Geometry check sheet. Reference: the model listing, model coordinates, mm. A direction names the side the tool comes from. Round coordinates to 2 decimals unless told otherwise and drop trailing zeros. Loops run counter-clockwise (first coordinate to the right, second up) from the corner with the lowest first, then second, coordinate; pieces in that order, holes last. Notation, with made-up numbers: M 55,37 L 91,37 A22 ccw 91,45 Z; hole C 10.5,25 d9. An arc over 180 degrees is marked long. Use one line per item in the form item = value. Start each with the question number.
1. Material ranges on line 1 (Z direction, x = -14, y = -122); line 2 (Z direction, x = -56, y = -116.5); line 3 (Z direction, x = 24.5, y = -119), recorded low to high.
2. Cross-section at C-C (z = 9.5). Record the boundary of the cut face in (x, y).
3. Cross-section at D-D (z = 34.5). Record the boundary of the cut face in (x, y).
4. Cross-section at B-B (y = -124). State how many separate pieces and enclosed holes the cut face has, then the cut area to 3 significant figures.
5. Go/stop test with flat-tipped pins: pin 1 (1 mm diameter, centred on x = 19, z = 45.5, fed in from +Y); pin 2 (10 mm diameter, centred on x = -14.5, z = 44.5, fed in from -Y); pin 3 (10 mm diameter, centred on x = -21, z = 31.5, fed in from -Y). Record where each tip stops, or that it passes through.
6. Cross-section at A-A (z = 44). Record the boundary of the cut face in (x, y), then the cut area to 3 significant figures.
7. Draft check along Z on faces 1 (the flat face through (-1, -124, 37.5)), 2 (the flat face through (-65.03, -108, 46)), 3 (the flat face through (-1, -116, 66)), 4 (the flat face through (-1, -112.1, 52)). Enter one of: pulls with the +Z half, pulls with the -Z half, needs draft (parallel to the pull), parting line crosses it, or undercut.
8. Set-up check for faces 5 (the flat face through (64.97, -108, 46)), 6 (the cylindrical face through (-0.995, -137.496, 38.966)), 7 (the flat face through (-1, -122, 40.46)), 8 (the cylindrical face through (-0.995, -122.496, 16.96)): record each of +Z, -Z, +X, -X, +Y, -Y from which the full face is reachable in a straight line by a thin tool's end or side.
```python
from build123d import *

# Parameters (mm, degrees)
BOX003_W      = 570
BOX003_H      = 100
BOX003_DEPTH  = 22.5
TUBE003_R     = 250
TUBE003_R_2   = 122.5
TUBE003_DEPTH = 37.5
TUBE002_R     = 250
TUBE002_R_2   = 122.5
TUBE002_DEPTH = 37.5
TUBE001_R     = 250
TUBE001_R_2   = 122.5
TUBE001_DEPTH = 40.5
BOX001_W      = 570
BOX001_H      = 100
BOX001_DEPTH  = 22.5
BOX_W         = 130
BOX_H         = 70
BOX_DEPTH     = 72
FILLET_R      = 1
FILLET001_R   = 0.5
FILLET002_R   = 0.5
FILLET003_R   = 0.5


with BuildPart() as sphere:
    # Sphere → Sphere (revolve)
    with BuildSketch(Plane(origin=(-0.01, -10.37, -8.39), x_dir=(1, 0, 0), z_dir=(0, -1, 0))):
        with BuildLine():
            ThreePointArc((0, -110), (110, 0), (0, 110))
            Line((0, 110), (0, -110))
        make_face()
    revolve(axis=Axis((-0.01, -10.37, -8.39), (0, 0, 1)))


with BuildPart() as box003:
    # Box003 → Box003 (new body)
    with BuildSketch(Plane(origin=(-285.31, -232.1, 44.4), x_dir=(1, 0, 0), z_dir=(0, 0, 1))):
        with Locations((285, 50)):
            Rectangle(BOX003_W, BOX003_H)
    extrude(amount=BOX003_DEPTH)


with BuildPart() as tube003:
    # Tube003 → Tube003 (new body)
    with BuildSketch(Plane(origin=(0, -15, 10), x_dir=(1, 0, 0), z_dir=(0, 0, 1))):
        Circle(TUBE003_R)
        Circle(TUBE003_R_2, mode=Mode.SUBTRACT)
    extrude(amount=TUBE003_DEPTH)


with BuildPart() as tube002:
    # Tube002 → Tube002 (new body)
    with BuildSketch(Plane(origin=(0, -5, -10), x_dir=(1, 0, 0), z_dir=(0, 0, 1))):
        Circle(TUBE002_R)
        Circle(TUBE002_R_2, mode=Mode.SUBTRACT)
    extrude(amount=TUBE002_DEPTH)


with BuildPart() as tube001:
    # Tube001 → Tube001 (new body)
    with BuildSketch(Plane.XY.offset(-3)):
        Circle(TUBE001_R)
        Circle(TUBE001_R_2, mode=Mode.SUBTRACT)
    extrude(amount=TUBE001_DEPTH)


with BuildPart() as box001:
    # Box001 → Box001 (new body)
    with BuildSketch(Plane(origin=(-285.31, -212.1, 40.46), x_dir=(1, 0, 0), z_dir=(0, 0, 1))):
        with Locations((285, 50)):
            Rectangle(BOX001_W, BOX001_H)
    extrude(amount=BOX001_DEPTH)


with BuildPart() as fillet003:
    # Box → Box (new body)
    with BuildSketch(Plane(origin=(-65.03, -170.42, -6), x_dir=(1, 0, 0), z_dir=(0, 0, 1))):
        with Locations((65, 35)):
            Rectangle(BOX_W, BOX_H)
    extrude(amount=BOX_DEPTH)

    # Cut: cut Box001
    add(box001.part, mode=Mode.SUBTRACT)

    # Cut001: cut Tube001
    add(tube001.part, mode=Mode.SUBTRACT)

    # Cut002: cut Tube002
    add(tube002.part, mode=Mode.SUBTRACT)

    # Cut003: cut Tube003
    add(tube003.part, mode=Mode.SUBTRACT)

    # Cut004: cut Box003
    add(box003.part, mode=Mode.SUBTRACT)

    # Cut005: cut Sphere
    add(sphere.part, mode=Mode.SUBTRACT)

    # Fillet
    fillet_edges = [fillet003.edges().sort_by_distance(p)[0] for p in [
        (-65.03, -100.42, 30),
        (-0.03, -100.42, 66),
        (-64.084558, -100.42, -6),
        (64.044558, -100.42, -6),
        (64.97, -100.42, 30),
        (-0.01, -120.344033, -6),
    ]]
    fillet(fillet_edges, radius=FILLET_R)

    # Fillet001
    fillet001_edges = [fillet003.edges().sort_by_distance(p)[0] for p in [
        (-65.03, -105.117006, -6),
        (64.97, -105.135786, -6),
    ]]
    fillet(fillet001_edges, radius=FILLET001_R)

    # Fillet002
    fillet002_edges = [fillet003.edges().sort_by_distance(p)[0] for p in [
        (-65.03, -111.314012, 37.5),
        (-65.03, -106.314012, -3),
        (-0.035393, -127.499995, -3),
        (64.97, -106.351572, -3),
        (64.97, -111.351572, 37.5),
        (-0.035393, -137.499995, 37.5),
    ]]
    fillet(fillet002_edges, radius=FILLET002_R)

    # Fillet003
    fillet003_edges = [fillet003.edges().sort_by_distance(p)[0] for p in [
        (-65.03, -116.76, 66),
        (-65.03, -122.1, 62.96),
        (-65.03, -112.1, 51.71),
        (-65.03, -115.457006, 40.46),
        (-0.03, -132.1, 66),
        (64.97, -116.76, 66),
        (-0.03, -132.1, 62.96),
        (64.97, -122.1, 62.96),
        (-0.035393, -137.499995, 40.46),
        (64.97, -112.1, 51.71),
        (64.97, -115.475786, 40.46),
    ]]
    fillet(fillet003_edges, radius=FILLET003_R)


solid = fillet003.part
```
Reported:
q1.line_1 = -6 to -3, 37.5 to 40.46, 62.96 to 66
q1.line_2 = 37.5 to 40.46, 62.96 to 66
q1.line_3 = -6 to 40.46, 62.96 to 66
q2.outline = M -65.03,-103.81 A122.5 ccw 64.97,-103.85 L 64.97,-101.42 A1 ccw 63.97,-100.42 L 60.58,-100.42 A108.54 cw -60.6,-100.42 L -64.03,-100.42 A1 ccw -65.03,-101.42 Z
q3.outline = M -65.03,-103.81 A122.5 ccw 64.97,-103.85 L 64.97,-101.42 A1 ccw 63.97,-100.42 L 46.37,-100.42 A101.29 cw -46.39,-100.42 L -64.03,-100.42 A1 ccw -65.03,-101.42 Z
q4.separate_pieces = 3
q4.enclosed_holes = 0
q4.area = 899 mm²
q5.pin_1 = -104.06
q5.pin_2 = -136.88
q5.pin_3 = -121.45
q6.outline = M -65.03,-111.6 A0.5 ccw -64.53,-112.1 L 64.47,-112.1 A0.5 ccw 64.97,-111.6 L 64.97,-101.42 A1 ccw 63.97,-100.42 L 35.29,-100.42 A96.72 cw -35.31,-100.42 L -64.03,-100.42 A1 ccw -65.03,-101.42 Z
q6.area = 1,200 mm²
q7.face_1 = undercut
q7.face_2 = needs draft
q7.face_3 = pulls with the +Z half
q7.face_4 = undercut
q8.face_5 = +Z, -Z, +X, +Y, -Y
q8.face_6 = -Z, -Y
q8.face_7 = +X, -X, -Y
q8.face_8 = -Y
